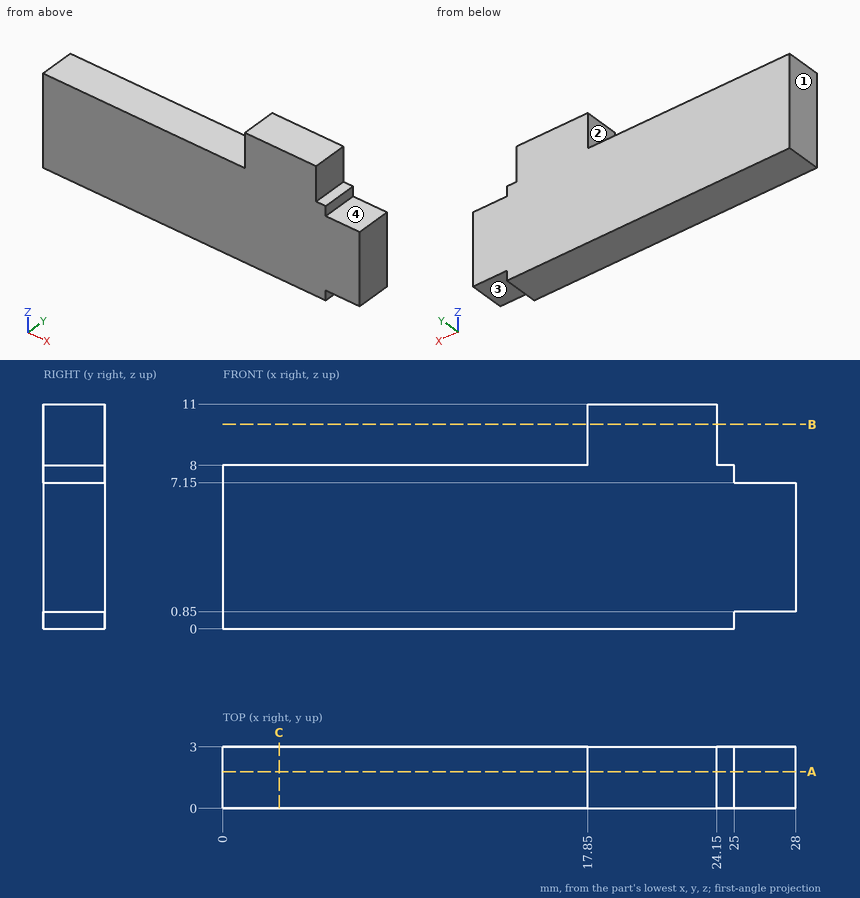
Can you work these out from the drawing? Everything is in mm from the part's minimum corner. A direction names the side the tool comes from. Coordinates: 2 decimals unless noted, no trailing zeros. Order: outer loops, then holes, each group sorted by start corner. A loop starts at its lowest first (then second) coordinate and runs counter-clockwise, first axis right, second up. Notation, with made-up numbers: (6, 84) -> (12, 84) arc R14 ccw to (12, 104) -> close; hole circle Ø7 at (-14, 69). An arc over 180 degrees is marked (long way). Return JSON: item names as keys, results as strings.
1) On a 3-axis mill with a long thin cutter (end or side, diameter ignored), from which of +Z, -Z, +X, -X, +Y, -Y can I reach the whole of each face in a straight line? I mean the marked faces 1, 2, 3 and 4. Say none if no direction works.
Conclusion:
{"face 1": "+Z, -Z, -X, +Y, -Y", "face 2": "+Z, -X, +Y, -Y", "face 3": "-Z, +X, +Y, -Y", "face 4": "+Z, +X, +Y, -Y"}
2) If we section it at A-A on y = 1.8: List the corners of the cut face in (x, z) for me, plus the area to 3 significant figures.
Conclusion:
{"outline": "(0, 0) -> (25, 0) -> (25, 0.85) -> (28, 0.85) -> (28, 7.15) -> (25, 7.15) -> (25, 8) -> (24.15, 8) -> (24.15, 11) -> (17.85, 11) -> (17.85, 8) -> (0, 8) -> close", "area": "238 mm²"}
3) I'm going to push flat-ended pins straight in: P1, Ø0.9, axis at x = 26, y = 2, coming from the +Z side; P2, Ø1.5, axis at y = 1.5, z = 9.5, coming from the +X side. Where does each tip first touch, or does it pass through?
Conclusion:
{"P1": "stops at z = 7.15", "P2": "stops at x = 24.15"}
4) If I drill on probe 1 along Z at (x, y) = (15, 2.4); probe 2 along Z at (x, y) = (26.5, 1); probe 3 along X at (y, z) = (1.7, 8.75), over which ranges is the centre line in solid material (lowest first)?
Conclusion:
{"probe 1": "z = 0 to 8", "probe 2": "z = 0.85 to 7.15", "probe 3": "x = 17.85 to 24.15"}
5) If we section it at B-B on z = 10: List the corners of the cut face in (x, y) for me, plus the area to 3 significant figures.
Conclusion:
{"outline": "(17.85, 0) -> (24.15, 0) -> (24.15, 3) -> (17.85, 3) -> close", "area": "18.9 mm²"}
6) If we section it at C-C on x = 2.75: List the corners of the cut face in (y, z) for me, plus the area to 3 significant figures.
Conclusion:
{"outline": "(0, 0) -> (3, 0) -> (3, 8) -> (0, 8) -> close", "area": "24.0 mm²"}
